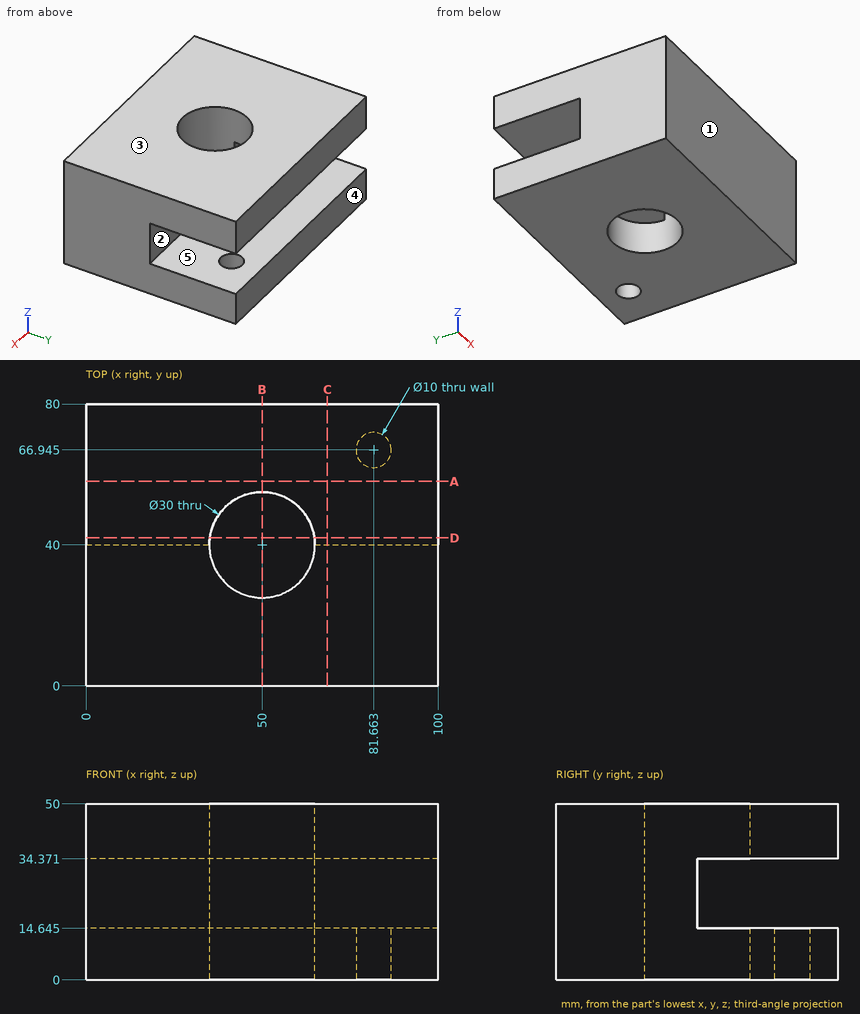
Print and shaded views of the part. All mm, measured from the part's lowest x, y and z. A direction names the side the tool comes from. Coordinates: 2 decimals unless noted, no trailing zeros. Loops run counter-clockwise (first coordinate to the right, second up) from the corner with the lowest first, then second, coordinate; pieces in that order, holes last. Notation, with made-up numbers: (59, -29) - (116, -29) arc R15 ccw to (116, -23) - close; hole circle Ø11 at (-0.75, -36). An arc over 180 degrees is marked (long way). Write item = value, one per line. Start each with the question number.
Item 1: Saw through at C-C, the plane x = 68.5. List the corners of the cut face in (y, z) (1 decimal), then the cut area to 3 significant figures.
Item 2: Saw through at D-D, the plane y = 42. List the corners of the cut face in (x, z) (1 decimal), then the cut area to 3 significant figures.
Item 3: Drop flat-ended pins along their axis: pin 1 Ø4 at (x, z) = (69, 18) entering from +Y; pin 2 Ø6 at (x, y) = (81.66, 66.94) entering from -Z. Give the stop position or say it passes through.
Item 4: 3-axis set-ups, long thin cutter, end or side, ignore diameter. For the marked faces 1 and 2: which of +Z, -Z, +X, -X, +Y, -Y reach the whole face in a straight line?
Item 5: Wall check: probe 1 along Z at (x, y) = (86.5, 60.5) (1 decimal); probe 2 along Y at (x, z) = (85.5, 28); probe 3 along Y at (x, z) = (50, 33). Give the ranges that are in metal, low to high. Write a range as [from, to].
Item 6: Saw through at A-A, the plane y = 58. List the corners of the cut face in (x, z) (1 decimal), then the cut area to 3 significant figures.
Item 7: Saw through at B-B, the plane x = 50. List the corners of the cut face in (y, z) (1 decimal).
Item 8: Pull direction Z, two halves, no side cores. Call the marked faces 3, 4 and 5: +Z half, -Z half, draft (parallel to the pull), parting line (faces both ways), or undercut.
Answers:
q1.outline = (0, 0) - (80, 0) - (80, 14.6) - (40, 14.6) - (40, 34.4) - (80, 34.4) - (80, 50) - (0, 50) - close
q1.area = 3,210 mm2
q2.outline = (0, 0) - (35.1, 0) - (35.1, 14.6) - (0, 14.6) - close; (0, 34.4) - (35.1, 34.4) - (35.1, 50) - (0, 50) - close; (64.9, 0) - (100, 0) - (100, 14.6) - (64.9, 14.6) - close; (64.9, 34.4) - (100, 34.4) - (100, 50) - (64.9, 50) - close
q2.area = 2,130 mm2
q3.pin_1 = 40
q3.pin_2 = 34.37
q4.face_1 = +Z, -Z, +X, -X, -Y
q4.face_2 = +X, -X, +Y
q5.probe_1 = [0, 14.6], [34.4, 50]
q5.probe_2 = [0, 40]
q5.probe_3 = [0, 25]
q6.outline = (0, 0) - (100, 0) - (100, 14.6) - (0, 14.6) - close; (0, 34.4) - (100, 34.4) - (100, 50) - (0, 50) - close
q6.area = 3,030 mm2
q7.outline = (0, 0) - (25, 0) - (25, 50) - (0, 50) - close; (55, 0) - (80, 0) - (80, 14.6) - (55, 14.6) - close; (55, 34.4) - (80, 34.4) - (80, 50) - (55, 50) - close
q8.face_3 = +Z half
q8.face_4 = draft
q8.face_5 = undercut
